```python
from build123d import *

# Parameters (mm, degrees)
SKETCH1_W           = 100
SKETCH1_H           = 100
SKETCH1_R           = 1.5
SKETCH1_R_2         = 3.5
BOSS_EXTRUDE1_DEPTH = 1.4
FILLET1_R           = 5


with BuildPart() as part:
    # Sketch1 → Boss-Extrude1 (new body)
    with BuildSketch(Plane(origin=(0, 0, 0), x_dir=(1, 0, 0), z_dir=(0, 1, 0))):
        Rectangle(SKETCH1_W, SKETCH1_H)
        with Locations(Location((-45.5, 45.5, 0), (0, 0, 270))):
            Circle(SKETCH1_R, mode=Mode.SUBTRACT)
        with Locations(Location((45.5, 45.5, 0), (0, 0, 270))):
            Circle(SKETCH1_R, mode=Mode.SUBTRACT)
        with Locations(Location((-45.5, -45.5, 0), (0, 0, 270))):
            Circle(SKETCH1_R, mode=Mode.SUBTRACT)
        with Locations(Location((45.5, -45.5, 0), (0, 0, 270))):
            Circle(SKETCH1_R, mode=Mode.SUBTRACT)
        with Locations(Location((0, 22, 0), (0, 0, 270))):
            Circle(SKETCH1_R_2, mode=Mode.SUBTRACT)
        with Locations(Location((0, -22, 0), (0, 0, 270))):
            Circle(SKETCH1_R_2, mode=Mode.SUBTRACT)
        with BuildLine():
            Line((-42.626255843, 36.25), (-42.626255843, -36.25))
            ThreePointArc((-42.626255843, -36.25), (-40.443668748, -38.940825635), (-37.360406683, -37.360406683))
            Line((-37.360406683, -37.360406683), (-37.360406683, 37.360406683))
            ThreePointArc((-37.360406683, 37.360406683), (-40.443668748, 38.940825635), (-42.626255843, 36.25))
        make_face(mode=Mode.SUBTRACT)
        with BuildLine():
            Line((-28, 39.8), (-28, 6.7))
            ThreePointArc((-28, 6.7), (-25.8, 4.5), (-23.6, 6.7))
            Line((-23.6, 6.7), (-23.6, 39.8))
            ThreePointArc((-23.6, 39.8), (-25.8, 42), (-28, 39.8))
        make_face(mode=Mode.SUBTRACT)
        with BuildLine():
            Line((-14.6, 39.8), (-14.6, 6.7))
            ThreePointArc((-14.6, 6.7), (-12.4, 4.5), (-10.2, 6.7))
            Line((-10.2, 6.7), (-10.2, 39.8))
            ThreePointArc((-10.2, 39.8), (-12.4, 42), (-14.6, 39.8))
        make_face(mode=Mode.SUBTRACT)
        with BuildLine():
            Line((-10.2, -39.8), (-10.2, -6.7))
            ThreePointArc((-10.2, -6.7), (-12.4, -4.5), (-14.6, -6.7))
            Line((-14.6, -6.7), (-14.6, -39.8))
            ThreePointArc((-14.6, -39.8), (-12.4, -42), (-10.2, -39.8))
        make_face(mode=Mode.SUBTRACT)
        with BuildLine():
            Line((-23.6, -39.8), (-23.6, -6.7))
            ThreePointArc((-23.6, -6.7), (-25.8, -4.5), (-28, -6.7))
            Line((-28, -6.7), (-28, -39.8))
            ThreePointArc((-28, -39.8), (-25.8, -42), (-23.6, -39.8))
        make_face(mode=Mode.SUBTRACT)
        with BuildLine():
            Line((10.2, -39.8), (10.2, -6.7))
            ThreePointArc((10.2, -6.7), (12.4, -4.5), (14.6, -6.7))
            Line((14.6, -6.7), (14.6, -39.8))
            ThreePointArc((14.6, -39.8), (12.4, -42), (10.2, -39.8))
        make_face(mode=Mode.SUBTRACT)
        with BuildLine():
            Line((10.2, 39.8), (10.2, 6.7))
            ThreePointArc((10.2, 6.7), (12.4, 4.5), (14.6, 6.7))
            Line((14.6, 6.7), (14.6, 39.8))
            ThreePointArc((14.6, 39.8), (12.4, 42), (10.2, 39.8))
        make_face(mode=Mode.SUBTRACT)
        with BuildLine():
            Line((23.6, -39.8), (23.6, -6.7))
            ThreePointArc((23.6, -6.7), (25.8, -4.5), (28, -6.7))
            Line((28, -6.7), (28, -39.8))
            ThreePointArc((28, -39.8), (25.8, -42), (23.6, -39.8))
        make_face(mode=Mode.SUBTRACT)
        with BuildLine():
            Line((23.6, 39.8), (23.6, 6.7))
            ThreePointArc((23.6, 6.7), (25.8, 4.5), (28, 6.7))
            Line((28, 6.7), (28, 39.8))
            ThreePointArc((28, 39.8), (25.8, 42), (23.6, 39.8))
        make_face(mode=Mode.SUBTRACT)
        with BuildLine():
            Line((37.360406683, 37.360406683), (37.360406683, -37.360406683))
            ThreePointArc((37.360406683, -37.360406683), (40.443668748, -38.940825635), (42.626255843, -36.25))
            Line((42.626255843, -36.25), (42.626255843, 36.25))
            ThreePointArc((42.626255843, 36.25), (40.443668748, 38.940825635), (37.360406683, 37.360406683))
        make_face(mode=Mode.SUBTRACT)
    extrude(amount=BOSS_EXTRUDE1_DEPTH)

    # Fillet1
    fillet1_edges = [part.edges().sort_by_distance(p)[0] for p in [
        (-50, 0.7, -50),
        (50, 0.7, -50),
        (50, 0.7, 50),
        (-50, 0.7, 50),
    ]]
    fillet(fillet1_edges, radius=FILLET1_R)


solid = part.part
```
Design review of the part built by this model. Coordinates are the model's own, in mm. Coordinates: 2 decimals unless noted, no trailing zeros. Order: outer loops, then holes, each group sorted by start corner. A loop starts at its lowest first (then second) coordinate and runs counter-clockwise, first axis right, second up.
1) Wall thickness on line 1 along X through (y, z) = (0.75, 45.5); line 2 along X through (y, z) = (0.15, -40); line 3 along Z through (x, y) = (27.5, 0.1): over which ranges is each line inside the solid? List them lowest first.
2) Take a section at D-D, the plane x = -12.4. Give the boundary of the cut face in (y, z).
3) Take a section at A-A, the plane z = -27. Give the boundary of the cut face in (x, y).
4) Take a section at C-C, the plane y = 1.05. State how many separate pieces and enclosed holes the cut face has, and give its area (3 significant figures).
5) Take a section at B-B, the plane x = 0. Give the boundary of the cut face in (y, z), and give its area (3 significant figures).
6) Mouldability with a two-part tool opening along X and no side actions: class faces 1 (the cylindrical face through (-49, 1, 48)), 2 (the flat face through (-1, 1.4, -1)), 3 (the cylindrical face through (-46.4, 0.7, 44.3)) as +X half, -X half, draft (parallel to the pull), parting line (faces both ways), or undercut.
Returned:
1. line 1: x = -49.97 to -47, -44 to 44, 47 to 49.97
1. line 2: x = -50 to -27.99, -23.61 to -14.59, -10.21 to 10.21, 14.59 to 23.61, 27.99 to 50
1. line 3: z = -50 to -41.2, -5.3 to 5.3, 41.2 to 50
2. outline: (0, -50) - (1.4, -50) - (1.4, -42) - (0, -42) - close; (0, -4.5) - (1.4, -4.5) - (1.4, 4.5) - (0, 4.5) - close; (0, 42) - (1.4, 42) - (1.4, 50) - (0, 50) - close
3. outline: (-50, 0) - (-42.63, 0) - (-42.63, 1.4) - (-50, 1.4) - close; (-37.36, 0) - (-28, 0) - (-28, 1.4) - (-37.36, 1.4) - close; (-23.6, 0) - (-14.6, 0) - (-14.6, 1.4) - (-23.6, 1.4) - close; (-10.2, 0) - (10.2, 0) - (10.2, 1.4) - (-10.2, 1.4) - close; (14.6, 0) - (23.6, 0) - (23.6, 1.4) - (14.6, 1.4) - close; (28, 0) - (37.36, 0) - (37.36, 1.4) - (28, 1.4) - close; (42.63, 0) - (50, 0) - (50, 1.4) - (42.63, 1.4) - close
4. separate pieces: 1
4. enclosed holes: 16
4. area: 7,780 mm2
5. outline: (0, -50) - (1.4, -50) - (1.4, -25.5) - (0, -25.5) - close; (0, -18.5) - (1.4, -18.5) - (1.4, 18.5) - (0, 18.5) - close; (0, 25.5) - (1.4, 25.5) - (1.4, 50) - (0, 50) - close
5. area: 120 mm2
6. face 1: -X half
6. face 2: draft
6. face 3: undercut
